Check sheet for the modelled part. Datum: model origin and axes. Units: mm. A direction names the side the tool comes from. Give positions to 0.01 mm unless a question says otherwise; leave off trailing zeros. Order: outer loops, then holes, each group sorted by start corner. A loop starts at its lowest first (then second) coordinate and runs counter-clockwise, first axis right, second up.
```python
from build123d import *

# Parameters (mm, degrees)
F0_R     = 7.6
F1_DEPTH = 100
F2_R     = 2.75
F3_DEPTH = 15
F4_R     = 3


with BuildPart() as f1:
    # F0 (on Right) → F1 (new body)
    with BuildSketch(Plane.YZ):
        with BuildLine():
            Line((0, 60), (0, 0))
            Line((0, 0), (60, 0))
            Line((60, 0), (60, 15))
            Line((60, 15), (38, 15))
            ThreePointArc((38, 15), (32.343146, 17.343146), (30, 23))
            Line((30, 23), (30, 60))
            Line((30, 60), (0, 60))
        make_face()
        with Locations((15, 45)):
            Circle(F0_R, mode=Mode.SUBTRACT)
    extrude(amount=F1_DEPTH)

    # F2 (on Top) → F3 (cut)
    with BuildSketch(Plane.XY):
        with Locations((15, 47.5)):
            Circle(F2_R)
        with Locations((85, 47.5)):
            Circle(F2_R)
    extrude(amount=F3_DEPTH, mode=Mode.SUBTRACT)

    # F4
    f4_edges = [f1.edges().sort_by_distance(p)[0] for p in [
        (100, 15, 60),
        (0, 15, 60),
        (50, 30, 60),
        (50, 0, 60),
        (100, 49, 15),
        (50, 60, 15),
        (0, 49, 15),
        (100, 0, 30),
        (0, 0, 30),
        (0, 60, 7.5),
        (100, 60, 7.5),
    ]]
    fillet(f4_edges, radius=F4_R)


solid = f1.part
```
(1) Release check for a two-part mould opening along Y. For faces 6 (the face through (0.9, 14.83, 59.14)), 7 (the face through (99.14, 29.1, 40.24)), 8 (the face through (49.3, 9.4, 50.14)), 9 (the face through (14.642, 50.227, 7.395)) record: released by +Y, released by -Y, zero draft, split by the parting line, or undercut.
Response values:
face 6: zero draft
face 7: released by +Y
face 8: undercut
face 9: undercut
(2) Material ranges on L1, parallel to Y at x = 15, z = 11; L2, parallel to Z at x = 51, y = 15; L3, parallel to Y at x = 41, z = 39.5 (3 decimals), recorded low to high.
Response values:
L1: y = 0 to 44.75, 50.25 to 60
L2: z = 0 to 37.4, 52.6 to 60
L3: y = 0 to 9.755, 20.245 to 30
(3) Cross-section at C-C on z = 45. Enter the section's corners in (x, y).
Response values:
outline: (0, 3) arc R3 ccw to (3, 0) - (97, 0) arc R3 ccw to (100, 3) - (100, 7.4) - (0, 7.4) - close; (0, 22.6) - (100, 22.6) - (100, 27) arc R3 ccw to (97, 30) - (3, 30) arc R3 ccw to (0, 27) - close
(4) Cross-section at B-B on x = 85. Enter the section's corners in (y, z).
Response values:
outline: (0, 0) - (44.75, 0) - (44.75, 15) - (38, 15) arc R8 cw to (30, 23) - (30, 57) arc R3 ccw to (27, 60) - (3, 60) arc R3 ccw to (0, 57) - close; (50.25, 0) - (60, 0) - (60, 12) arc R3 ccw to (57, 15) - (50.25, 15) - close; hole circle Ø15.2 at (15, 45)
(5) Gauge pin test, flat ends, axial feed: pin 1 Ø12 at (x, y) = (37, 39) entering from +Z (3 decimals); pin 2 Ø15 at (x, y) = (67, 52) entering from +Z; pin 3 Ø1.5 at (x, z) = (63, 50) entering from +Y. Record the tip position at first contact, or that the pin passes through.
Response values:
pin 1: stops at z = 16.755
pin 2: stops at z = 15
pin 3: stops at y = 30
(6) Cross-section at D-D on x = 23. Enter the section's corners in (y, z), then the cut area to 3 significant figures.
Response values:
outline: (0, 0) - (60, 0) - (60, 12) arc R3 ccw to (57, 15) - (38, 15) arc R8 cw to (30, 23) - (30, 57) arc R3 ccw to (27, 60) - (3, 60) arc R3 ccw to (0, 57) - close; hole circle Ø15.2 at (15, 45)
area: 2,080 mm2
(7) Cross-section at A-A on y = 47.5. Enter the section's corners in (x, z).
Response values:
outline: (0, 0) - (12.25, 0) - (12.25, 15) - (3, 15) arc R3 ccw to (0, 12) - close; (17.75, 0) - (82.25, 0) - (82.25, 15) - (17.75, 15) - close; (87.75, 0) - (100, 0) - (100, 12) arc R3 ccw to (97, 15) - (87.75, 15) - close
(8) Set-up check for faces 1 (the face through (49, 30, 40)), 2 (the face through (99.14, 47.37, 14.1)), 3 (the face through (100, 24, 23)), 4 (the face through (0.86, 47.37, 14.1)), 5 (the face through (99.1, 14.83, 59.14)): record each of +Z, -Z, +X, -X, +Y, -Y from which the full face is reachable in a straight line by a thin tool's end or side.
Response values:
face 1: +Z, +X, -X, +Y
face 2: +Z, +X, +Y
face 3: +Z, -Z, +X, +Y, -Y
face 4: +Z, -X, +Y
face 5: +Z, +X, +Y, -Y
